from build123d import *

# Parameters (mm, degrees)
SKETCH1_W           = 13
SKETCH1_H           = 10
BOSS_EXTRUDE1_DEPTH = 2
SKETCH2_W           = 2
SKETCH2_H           = 10
BOSS_EXTRUDE2_DEPTH = 25
SKETCH4_W           = 2
SKETCH4_H           = 25
BOSS_EXTRUDE3_DEPTH = 7.5
SKETCH5_W           = 2
SKETCH5_H           = 25
BOSS_EXTRUDE4_DEPTH = 7.5
SKETCH6_R           = 2
CUT_EXTRUDE1_DEPTH  = 7.5
SKETCH7_R           = 9.5
CUT_EXTRUDE2_DEPTH  = 32.721443851


with BuildPart() as part:
    # Sketch1 → Boss-Extrude1 (new body)
    with BuildSketch(Plane.XY):
        Rectangle(SKETCH1_W, SKETCH1_H)
    extrude(amount=BOSS_EXTRUDE1_DEPTH)

    # Sketch2 → Boss-Extrude2 (add)
    with BuildSketch(Plane.XY.offset(2)):
        with Locations((-5.5, 0)):
            Rectangle(SKETCH2_W, SKETCH2_H)
    extrude(amount=BOSS_EXTRUDE2_DEPTH)

    # Sketch4 → Boss-Extrude3 (add)
    with BuildSketch(Plane(origin=(0, 5, 0), x_dir=(1, 0, 0), z_dir=(0, 1, 0))):
        with Locations((-5.5, -14.5)):
            Rectangle(SKETCH4_W, SKETCH4_H)
    extrude(amount=BOSS_EXTRUDE3_DEPTH)

    # Sketch5 → Boss-Extrude4 (add)
    with BuildSketch(Plane.XZ.offset(5)):
        with Locations((-5.5, 14.5)):
            Rectangle(SKETCH5_W, SKETCH5_H)
    extrude(amount=BOSS_EXTRUDE4_DEPTH)

    # Sketch6 → Cut-Extrude1 (cut)
    with BuildSketch(Plane(origin=(0, 0, 0), x_dir=(-1, 0, 0), z_dir=(0, 0, -1))):
        Circle(SKETCH6_R)
    extrude(amount=-CUT_EXTRUDE1_DEPTH, mode=Mode.SUBTRACT)

    # Sketch7 → Cut-Extrude2 (cut, through all)
    with BuildSketch(Plane(origin=(-4.5, 0, 0), x_dir=(0, 0, -1), z_dir=(1, 0, 0))):
        with Locations(Location((-14.5, 0, 0), (0, 0, 90))):
            Circle(SKETCH7_R)
    extrude(amount=-CUT_EXTRUDE2_DEPTH, mode=Mode.SUBTRACT)


solid = part.part
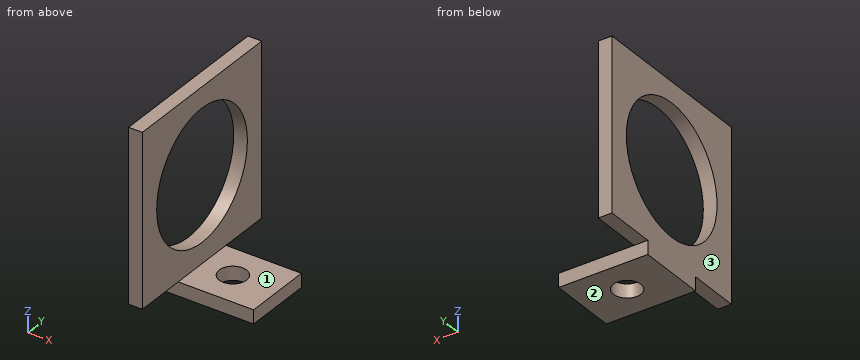
Input: part model. Units: mm. Frame: model coordinates. Face numbers are marked on the shaded views. Coordinates: 2 decimals unless noted, no trailing zeros. Write each loop counter-clockwise with the first axis right and the second up, starting at its lowest first coordinate (ties: lowest second). Pieces come first, ordered by that corner, then holes. Notation, with made-up numbers: M -6.75,72.5 L 14.25,72.5 A24 ccw 14.25,105.5 Z; hole C 37,63.25 d6. An arc over 180 degrees is marked long. Answer as a JSON object with one key per item and string values. Group by question number.
(1) Ray query, line 1 along Y through (x, z) = (0, 1.5); line 2 along Z through (x, y) = (-5.45, 0); line 3 along X through (y, z) = (-11, 21.5). Return the intervals inside material, ascending. Write a range as [from, to].
(2) Section A-A on z = 14.5. Output: boundary loops of the cut face in (x, y).
(3) Contact query for flat-ended pins moving along their axis: P1, Ø1.6, axis at x = 2, z = 1, coming from the +Y side; P2, Ø1.6, axis at x = -5.5, y = -8, coming from the -Z side; P3, Ø1, axis at x = 1, z = 1.5, coming from the -Y side. Output: stop coordinate, or through.
(4) Mould query, pull axis Z, two halves, no side actions, for the marked faces 1, 2 and 3. Classes: pulls with the +Z half, pulls with the -Z half, needs draft (parallel to the pull), parting line crosses it, or undercut.
(5) Section C-C on y = 0. Output: boundary loops of the cut face in (x, z), plus the area to 3 significant figures.
(6) Section D-D on x = -5.25. Output: boundary loops of the cut face in (y, z), plus the area to 3 significant figures.
(7) Section B-B on x = 0. Output: boundary loops of the cut face in (y, z).
Result set:
{
 "1": {"line 1": "y = [-5, -2], [2, 5]", "line 2": "z = [0, 5], [24, 27]", "line 3": "x = [-6.5, -4.5]"},
 "2": {"outline": "M -6.5,-12.5 L -4.5,-12.5 L -4.5,-9.5 L -6.5,-9.5 Z; M -6.5,9.5 L -4.5,9.5 L -4.5,12.5 L -6.5,12.5 Z"},
 "3": {"P1": "stops at y = 5", "P2": "stops at z = 2", "P3": "stops at y = -5"},
 "4": {"face 1": "pulls with the +Z half", "face 2": "pulls with the -Z half", "face 3": "needs draft"},
 "5": {"outline": "M -6.5,0 L -2,0 L -2,2 L -4.5,2 L -4.5,5 L -6.5,5 Z; M -6.5,24 L -4.5,24 L -4.5,27 L -6.5,27 Z; M 2,0 L 6.5,0 L 6.5,2 L 2,2 Z", "area": "30.0 mm2"},
 "6": {"outline": "M -12.5,2 L -5,2 L -5,0 L 5,0 L 5,2 L 12.5,2 L 12.5,27 L -12.5,27 Z; hole C 0,14.5 d19", "area": "361 mm2"},
 "7": {"outline": "M -5,0 L -2,0 L -2,2 L -5,2 Z; M 2,0 L 5,0 L 5,2 L 2,2 Z"}
}
